Design review of the part built by this model. Coordinates are the model's own, in mm. A direction names the side the tool comes from. Round coordinates to 2 decimals unless told otherwise and drop trailing zeros. Order: outer loops, then holes, each group sorted by start corner. A loop starts at its lowest first (then second) coordinate and runs counter-clockwise, first axis right, second up. Notation, with made-up numbers: (65, -39.75) - (74, -39.75) arc R24 ccw to (74, -18.75) - close; hole circle Ø3 at (84, 47). An arc over 180 degrees is marked (long way). Write item = value, one per line.
from build123d import *

# Parameters (mm, degrees)
F0_R     = 10
F1_DEPTH = 25
F2_DEPTH = 50
F3_SIZE  = 2
F5_R     = 29.820432
F6_DEPTH = 25


with BuildPart() as f1:
    # F0 (on Front) → F1 (new body)
    with BuildSketch(Plane.XZ):
        with BuildLine():
            ThreePointArc((2.083333, -24.913043), (18.399502, -16.92508), (25, 0))
            ThreePointArc((25, 0), (18.399502, 16.92508), (2.083333, 24.913043))
            ThreePointArc((2.083333, 24.913043), (-25, 0), (2.083333, -24.913043))
        make_face()
        Circle(F0_R, mode=Mode.SUBTRACT)
        with BuildLine():
            ThreePointArc((2.083333, 24.913043), (18.399502, 16.92508), (25, 0))
            ThreePointArc((25, 0), (18.399502, -16.92508), (2.083333, -24.913043))
            Line((2.083333, -24.913043), (91.458333, -17.43913))
            ThreePointArc((91.458333, -17.43913), (72.5, 0), (91.458333, 17.43913))
            Line((91.458333, 17.43913), (2.083333, 24.913043))
        make_face()
        with BuildLine():
            ThreePointArc((107.5, 0), (102.879651, 11.847556), (91.458333, 17.43913))
            ThreePointArc((91.458333, 17.43913), (72.5, 0), (91.458333, -17.43913))
            ThreePointArc((91.458333, -17.43913), (102.879651, -11.847556), (107.5, 0))
        make_face()
        with Locations((90, 0)):
            Circle(F0_R, mode=Mode.SUBTRACT)
    extrude(amount=F1_DEPTH)

    # F0 (on Front) → F2 (join)
    with BuildSketch(Plane.XZ):
        with BuildLine():
            ThreePointArc((2.083333, -24.913043), (18.399502, -16.92508), (25, 0))
            ThreePointArc((25, 0), (18.399502, 16.92508), (2.083333, 24.913043))
            ThreePointArc((2.083333, 24.913043), (-25, 0), (2.083333, -24.913043))
        make_face()
        Circle(F0_R, mode=Mode.SUBTRACT)
    extrude(amount=F2_DEPTH)

    # F3
    f3_edges = [f1.edges().sort_by_distance(p)[0] for p in [
        (-2.083333, -50, 24.913043),
        (-10, -50, 0),
        (80, -25, 0),
    ]]
    chamfer(f3_edges, length=F3_SIZE)

    # F0 (on Front) + F5 (on face) → F6 (join)
    with BuildSketch(Plane.XZ):
        with BuildLine():
            ThreePointArc((2.083333, -24.913043), (18.399502, -16.92508), (25, 0))
            ThreePointArc((25, 0), (18.399502, 16.92508), (2.083333, 24.913043))
            ThreePointArc((2.083333, 24.913043), (-25, 0), (2.083333, -24.913043))
        make_face()
        Circle(F0_R, mode=Mode.SUBTRACT)
        with BuildLine():
            ThreePointArc((2.083333, 24.913043), (18.399502, 16.92508), (25, 0))
            ThreePointArc((25, 0), (18.399502, -16.92508), (2.083333, -24.913043))
            Line((2.083333, -24.913043), (91.458333, -17.43913))
            ThreePointArc((91.458333, -17.43913), (72.5, 0), (91.458333, 17.43913))
            Line((91.458333, 17.43913), (2.083333, 24.913043))
        make_face()
        with BuildLine():
            ThreePointArc((107.5, 0), (102.879651, 11.847556), (91.458333, 17.43913))
            ThreePointArc((91.458333, 17.43913), (72.5, 0), (91.458333, -17.43913))
            ThreePointArc((91.458333, -17.43913), (102.879651, -11.847556), (107.5, 0))
        make_face()
        with Locations((90, 0)):
            Circle(F0_R, mode=Mode.SUBTRACT)
    with BuildSketch(Plane.XZ):
        with Locations((26.628146, 23.54129)):
            Circle(F5_R)
    extrude(amount=F6_DEPTH)


solid = f1.part
Item 1: Insertion check: P1, Ø2, axis at x = 76, z = -5.5, coming from the -Y side; P2, Ø6, axis at x = 9, y = -28.5, coming from the -Z side. Each pin has a flat end and moves straight along its axis. Give the tip position at first contact, or say it passes through.
Data:
P1 = -25
P2 = -24.27
Item 2: For line 1 along X through (y, z) = (-26, 0); line 2 along X through (y, z) = (-22.5, 8); line 3 along Y through (x, z) = (44, -21), list the stretches that pass through material, from the lowest coordinate up. Write a range as [from, to].
Data:
line_1 = [-25, -10], [10, 25]
line_2 = [-23.69, -6], [1.18, 84], [96, 105.56]
line_3 = [-25, 0]
Item 3: Take a section at A-A, the plane x = 90. State the section outline as (y, z) points, and give its area (3 significant figures).
Data:
outline = (-25, -17.56) - (0, -17.56) - (0, -10) - (-25, -10) - close; (-25, 10) - (0, 10) - (0, 17.56) - (-25, 17.56) - close
area = 378 mm2
Item 4: The part is to be moulded in two halves that separate along Z. For faces 4 (the face through (51, -25, 15)), 5 (the face through (46.15, -12.32, -21.23)), 6 (the face through (80, -12, 0)), say which applies: +Z half, -Z half, draft (parallel to the pull), parting line (faces both ways), or undercut.
Data:
face_4 = draft
face_5 = -Z half
face_6 = undercut
Item 5: Take a section at C-C, the plane y = -23.5. State the section outline as (x, z) points, and give its area (3 significant figures).
Data:
outline = (-3.17, 24.8) arc R25 ccw to (2.08, -24.91) - (91.46, -17.44) arc R17.5 ccw to (91.46, 17.44) - (56.28, 20.38) arc R29.82 ccw (long way) to start; hole (0.06, 10) arc R10 ccw (long way) to (9.93, -1.17) arc R29.82 cw to start; hole circle Ø20 at (90, 0)
area = 6,150 mm2
Item 6: For faces 1 (the face through (4.217, -12.325, 3.869)), 2 (the face through (6, -25, 4)), 3 (the face through (10, -50, -10)), list the 3-axis set-ups (+Z, -Z, +X, -X, +Y, -Y) from which the entire face can be reached by the end or side of a thin tool; tool diameter is ignored.
Data:
face_1 = +Y, -Y
face_2 = -Y
face_3 = +Z, -Z, +X, -X, -Y
Item 7: Take a section at D-D, the plane z = 2.5. Count the separate pieces of the cut face and the enclosed holes in it, and give its area (3 significant figures).
Data:
separate_pieces = 3
enclosed_holes = 0
area = 3,190 mm2
Item 8: Take a section at B-B, the plane y = -41. State the section outline as (x, z) points.
Data:
outline = (2.08, -24.91) arc R25 ccw to (25, 0) arc R25 ccw to (2.08, 24.91) arc R25 ccw (long way) to start; hole circle Ø20 at (0, 0)
